Job drawing, mm, ordinate dimensions from the low corner. One solid piece. Give positions to 0.01 mm unless a question says otherwise; leave off trailing zeros. Write each loop counter-clockwise with the first axis right and the second up, starting at its lowest first coordinate (ties: lowest second). Pieces come first, ordered by that corner, then holes. Notation, with made-up numbers: (76.25, -11) -> (103.25, -11) arc R28 ccw to (103.25, 12) -> close; hole circle Ø5 at (-29, 87.5). An arc over 180 degrees is marked (long way). One line per question, with ' | ' between items. Start each with the question number.
(1) Band-saw the part on A-A, the plane y = 20. Give the cut face in (x, z), and give its area (3 significant figures).
(2) Pull direction X, two halves, no side cores. Call the marked faces 1, 2, 3 and 4: released by +X, released by -X, zero draft, split by the parting line, or undercut.
(3) Drill centre lines: probe 1 along X at (y, z) = (14.5, 1.5); probe 2 along Y at (x, z) = (36, 16); probe 3 along Y at (x, z) = (52.5, 4.5). Where is each one in solid material? Low to high. Write a range as from..to.
(4) Band-saw the part on B-B, the plane x = 34.5. Give the cut face in (y, z).
(5) Pin check, flat tips, straight feed: P1, Ø4, axis at y = 28, z = 12.5, coming from the -X side; P2, Ø1.2, axis at x = 26.5, z = 4.5, coming from the +Y side; P3, Ø2.5, axis at x = 26.5, z = 20.5, coming from the +Y side; P4, Ø1.6, axis at y = 28, z = 20.5, coming from the +X side. Stop position of each tip, or through.
(6) Band-saw the part on C-C, the plane z = 9.25. Give the cut face in (x, y).
(7) Band-saw the part on D-D, the plane y = 38. Give the cut face in (x, z).
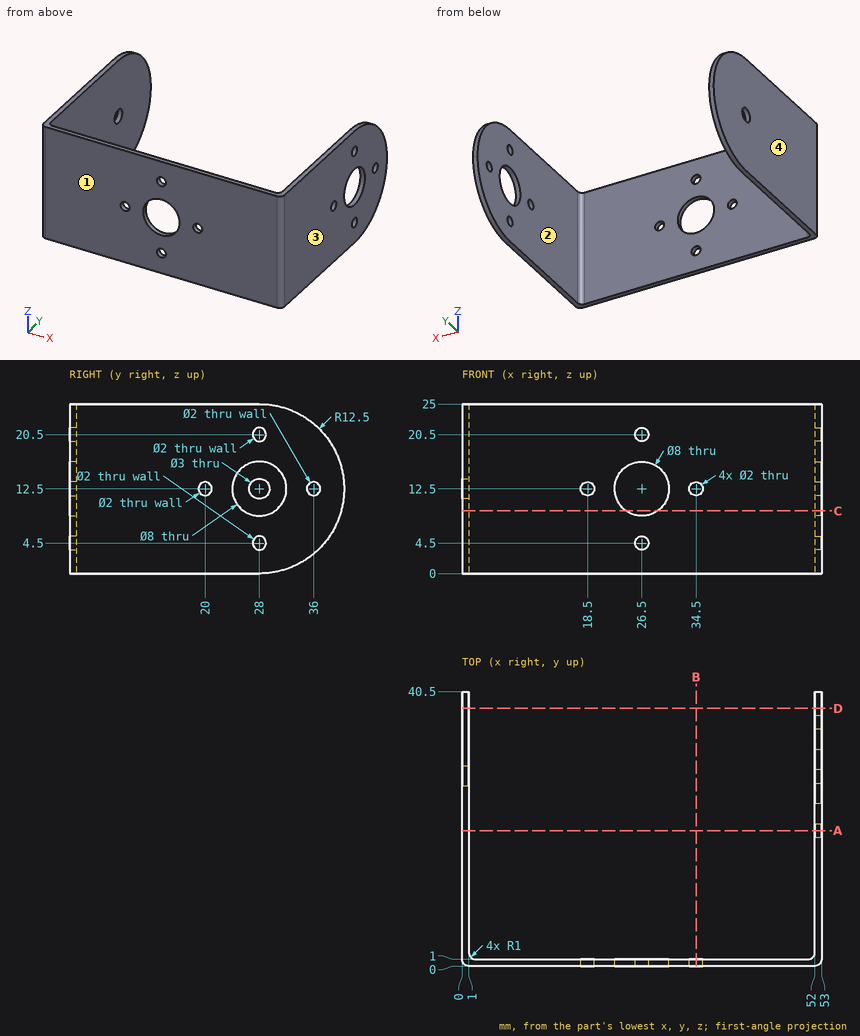
Results:
1) outline: (0, 0) -> (1, 0) -> (1, 25) -> (0, 25) -> close; (52, 0) -> (53, 0) -> (53, 11.5) -> (52, 11.5) -> close; (52, 13.5) -> (53, 13.5) -> (53, 25) -> (52, 25) -> close | area: 48.0 mm²
2) face 1: zero draft | face 2: undercut | face 3: released by +X | face 4: released by -X
3) probe 1: x = 0..1, 52..53 | probe 2: y = 0..1 | probe 3: y = 0.13..27, 29..37.6
4) outline: (0, 0) -> (1, 0) -> (1, 11.5) -> (0, 11.5) -> close; (0, 13.5) -> (1, 13.5) -> (1, 25) -> (0, 25) -> close
5) P1: stops at x = 0 | P2: passes through | P3: stops at y = 1 | P4: stops at x = 1
6) outline: (0, 1) arc R1 ccw to (1, 0) -> (24.17, 0) -> (24.17, 1) -> (2, 1) arc R1 cw to (1, 2) -> (1, 40.07) -> (0, 40.07) -> close; (28.83, 0) -> (52, 0) arc R1 ccw to (53, 1) -> (53, 25.67) -> (52, 25.67) -> (52, 2) arc R1 cw to (51, 1) -> (28.83, 1) -> close; (52, 30.33) -> (53, 30.33) -> (53, 40.07) -> (52, 40.07) -> close
7) outline: (0, 5) -> (1, 5) -> (1, 20) -> (0, 20) -> close; (52, 5) -> (53, 5) -> (53, 20) -> (52, 20) -> close
